Answer from the drawing. Dimensions are ordinates in mm from the lowest x, y and z of the part. A direction names the side the tool comes from. Round coordinates to 2 decimals unless told otherwise and drop trailing zeros. Write each loop counter-clockwise with the first axis right and the second up, starting at its lowest first coordinate (ties: lowest second). Pieces come first, ordered by that corner, then holes. Notation, with made-up numbers: (26, -21.75) -> (72, -21.75) arc R21 cw to (72, 17.25) -> close; hole circle Ø5 at (48, 11.5). An arc over 180 degrees is marked (long way). Answer as a JSON object with one key per item and string values. Group by question number.
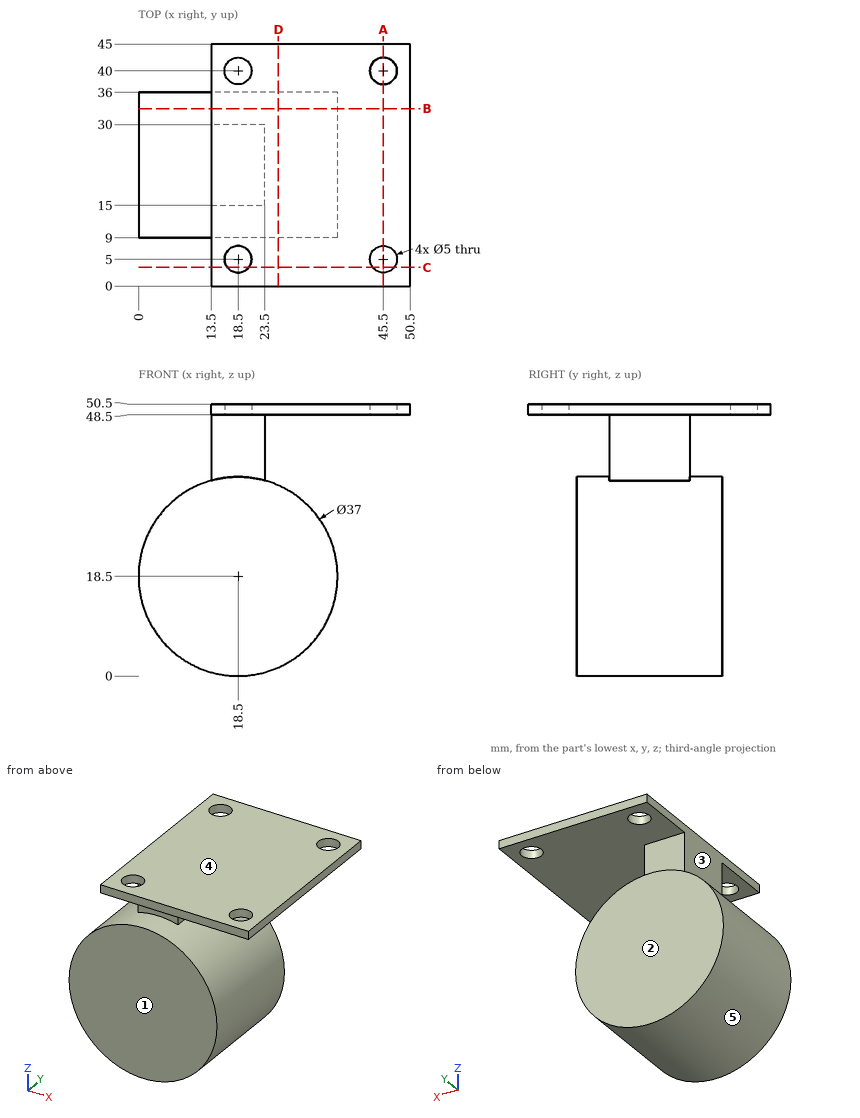
1) A cutting plane is placed at A-A on x = 45.5. Determine the outline of the cut face in (y, z), plus the area to 3 significant figures.
2) A tool of negligible diameter and unlimited length cuts with its end or side. For the marked faces 1 and 2, from which of +Z, -Z, +X, -X, +Y, -Y can it reach the whole face along a straight path? Write none if from no direction.
3) Straight lines are drawn through the part: L1, parallel to X at y = 40, z = 49; L2, parallel to Y at x = 18.5, z = 49.65; L3, parallel to Z at x = 31, y = 2.5. For each, find the intervals that lie inside material, in ascending order.
4) A cutting plane is placed at C-C on y = 3.5. Determine the outline of the cut face in (x, z).
5) A cutting plane is placed at B-B on y = 33. Determine the outline of the cut face in (x, z), plus the area to 3 significant figures.
6) Each of these flat-tipped pins is pushed along its axis until it touches: P1, Ø3, axis at y = 31, z = 28, coming from the -X side; P2, Ø8, axis at x = 26.5, z = 10.5, coming from the +Y side; P3, Ø7, axis at y = 15.5, z = 44, coming from the -X side. Where does it stop, or does it pass through?
7) A cutting plane is placed at D-D on x = 26. Determine the outline of the cut face in (y, z), plus the area to 3 significant figures.
8) For a pull along Z with two mould halves and no side action, classify the marked faces 3, 4 and 5 as released by +Z, released by -Z, zero draft, split by the parting line, or undercut.
Established:
{
 "1": {"outline": "(0, 48.5) -> (2.5, 48.5) -> (2.5, 50.5) -> (0, 50.5) -> close; (7.5, 48.5) -> (37.5, 48.5) -> (37.5, 50.5) -> (7.5, 50.5) -> close; (42.5, 48.5) -> (45, 48.5) -> (45, 50.5) -> (42.5, 50.5) -> close", "area": "70.0 mm²"},
 "2": {"face 1": "-Z, +X, -X, -Y", "face 2": "-Z, +X, -X, +Y"},
 "3": {"L1": "x = 13.5 to 16, 21 to 43, 48 to 50.5", "L2": "y = 0 to 2.5, 7.5 to 37.5, 42.5 to 45", "L3": "z = 48.5 to 50.5"},
 "4": {"outline": "(13.5, 48.5) -> (16.5, 48.5) -> (16.5, 50.5) -> (13.5, 50.5) -> close; (20.5, 48.5) -> (43.5, 48.5) -> (43.5, 50.5) -> (20.5, 50.5) -> close; (47.5, 48.5) -> (50.5, 48.5) -> (50.5, 50.5) -> (47.5, 50.5) -> close"},
 "5": {"outline": "circle Ø37 at (18.5, 18.5); (13.5, 48.5) -> (50.5, 48.5) -> (50.5, 50.5) -> (13.5, 50.5) -> close", "area": "1,150 mm²"},
 "6": {"P1": "stops at x = 1.82", "P2": "stops at y = 36", "P3": "stops at x = 13.5"},
 "7": {"outline": "(0, 48.5) -> (45, 48.5) -> (45, 50.5) -> (0, 50.5) -> close; (9, 1.59) -> (36, 1.59) -> (36, 35.41) -> (9, 35.41) -> close", "area": "1,000 mm²"},
 "8": {"face 3": "zero draft", "face 4": "released by +Z", "face 5": "undercut"}
}
